from build123d import *

# Parameters (mm, degrees)
SKETCH_2_W           = 57
SKETCH_2_H           = 47.14
EXTRUDE_1_DEPTH      = 100
SKETCH_3_R           = 17.5
EXTRUDE_2_DEPTH      = 2
SKETCH_4_R           = 5
EXTRUDE_3_DEPTH      = 22
SKETCH_5_W           = 15.396782634
SKETCH_5_H           = 5.477116352
CUT_EXTRUDE_1_DEPTH  = 20
SKETCH_7_R           = 10
CUT_EXTRUDE_2_DEPTH  = 95
SKETCH_8_R           = 2.5
CUT_EXTRUDE_3_DEPTH  = 90
SKETCH_9_OUTSIDE_W   = 87.878
SKETCH_9_OUTSIDE_H   = 78.018
SKETCH_9_OUTSIDE_W_2 = 55
SKETCH_9_OUTSIDE_H_2 = 47.14
CUT_EXTRUDE_4_DEPTH  = 80
CUT_EXTRUDE_5_DEPTH  = 40
CUT_EXTRUDE_6_DEPTH  = 20
SKETCH_12_R          = 2
CUT_EXTRUDE_7_DEPTH  = 4


with BuildPart() as part:
    # 草图2 → 凸台-拉伸1 (new body)
    with BuildSketch(Plane.XY):
        Rectangle(SKETCH_2_W, SKETCH_2_H)
    extrude(amount=EXTRUDE_1_DEPTH)

    # 草图3 → 凸台-拉伸2 (add)
    with BuildSketch(Plane.XY.offset(100)):
        Circle(SKETCH_3_R)
    extrude(amount=EXTRUDE_2_DEPTH)

    # 草图4 → 凸台-拉伸3 (add)
    with BuildSketch(Plane.XY.offset(102)):
        Circle(SKETCH_4_R)
    extrude(amount=EXTRUDE_3_DEPTH)

    # 草图5 → 切除-拉伸1 (cut)
    with BuildSketch(Plane.XY.offset(124)):
        with Locations((0.517283211, -5.738558176)):
            Rectangle(SKETCH_5_W, SKETCH_5_H)
    extrude(amount=-CUT_EXTRUDE_1_DEPTH, mode=Mode.SUBTRACT)

    # 草图7 → 切除-拉伸2 (cut)
    with BuildSketch(Plane(origin=(0, 0, 0), x_dir=(-1, 0, 0), z_dir=(0, 0, -1))):
        with Locations((28.5, 23.57)):
            Circle(SKETCH_7_R)
        with Locations((28.5, -23.57)):
            Circle(SKETCH_7_R)
        with Locations((-28.5, -23.57)):
            Circle(SKETCH_7_R)
        with Locations((-28.5, 23.57)):
            Circle(SKETCH_7_R)
    extrude(amount=-CUT_EXTRUDE_2_DEPTH, mode=Mode.SUBTRACT)

    # 草图8 → 切除-拉伸3 (cut)
    with BuildSketch(Plane.XY.offset(100)):
        with Locations((-24.5, 19.57)):
            Circle(SKETCH_8_R)
        with Locations((24.5, 19.57)):
            Circle(SKETCH_8_R)
        with Locations((24.5, -19.57)):
            Circle(SKETCH_8_R)
        with Locations((-24.5, -19.57)):
            Circle(SKETCH_8_R)
    extrude(amount=-CUT_EXTRUDE_3_DEPTH, mode=Mode.SUBTRACT)

    # 草图9 outside → 切除-拉伸4 (cut)
    with BuildSketch(Plane(origin=(0, 0, 0), x_dir=(-1, 0, 0), z_dir=(0, 0, -1))):
        Rectangle(SKETCH_9_OUTSIDE_W, SKETCH_9_OUTSIDE_H)
        Rectangle(SKETCH_9_OUTSIDE_W_2, SKETCH_9_OUTSIDE_H_2, mode=Mode.SUBTRACT)
    extrude(amount=-CUT_EXTRUDE_4_DEPTH, mode=Mode.SUBTRACT)

    # 草图10 → 切除-拉伸5 (cut)
    with BuildSketch(Plane(origin=(0, 0, 0), x_dir=(-1, 0, 0), z_dir=(0, 0, -1))):
        with BuildLine():
            Line((-27.5, 13.620125629), (-27.5, -13.620125629))
            ThreePointArc((-27.5, -13.620125629), (-21.083801513, -16.861796068), (-18.5, -23.57))
            Line((-18.5, -23.57), (18.5, -23.57))
            ThreePointArc((18.5, -23.57), (21.083801513, -16.861796068), (27.5, -13.620125629))
            Line((27.5, -13.620125629), (27.5, 13.620125629))
            ThreePointArc((27.5, 13.620125629), (21.083801513, 16.861796068), (18.5, 23.57))
            Line((18.5, 23.57), (-18.5, 23.57))
            ThreePointArc((-18.5, 23.57), (-21.083801513, 16.861796068), (-27.5, 13.620125629))
        make_face()
        with BuildLine():
            Line((-27, 13.177695155), (-27, -13.177695155))
            ThreePointArc((-27, -13.177695155), (-20.728707305, -16.509050358), (-18.011911518, -23.07))
            Line((-18.011911518, -23.07), (18.011911518, -23.07))
            ThreePointArc((18.011911518, -23.07), (20.728707305, -16.509050358), (27, -13.177695155))
            Line((27, -13.177695155), (27, 13.177695155))
            ThreePointArc((27, 13.177695155), (20.728707305, 16.509050358), (18.011911518, 23.07))
            Line((18.011911518, 23.07), (-18.011911518, 23.07))
            ThreePointArc((-18.011911518, 23.07), (-20.728707305, 16.509050358), (-27, 13.177695155))
        make_face(mode=Mode.SUBTRACT)
    extrude(amount=-CUT_EXTRUDE_5_DEPTH, mode=Mode.SUBTRACT)

    # 草图11 → 切除-拉伸6 (cut)
    with BuildSketch(Plane(origin=(0, 0, 0), x_dir=(-1, 0, 0), z_dir=(0, 0, -1))):
        with BuildLine():
            Line((-27, 13.177695155), (-27, -13.177695155))
            ThreePointArc((-27, -13.177695155), (-20.728707305, -16.509050358), (-18.011911518, -23.07))
            Line((-18.011911518, -23.07), (18.011911518, -23.07))
            ThreePointArc((18.011911518, -23.07), (20.728707305, -16.509050358), (27, -13.177695155))
            Line((27, -13.177695155), (27, 13.177695155))
            ThreePointArc((27, 13.177695155), (20.728707305, 16.509050358), (18.011911518, 23.07))
            Line((18.011911518, 23.07), (-18.011911518, 23.07))
            ThreePointArc((-18.011911518, 23.07), (-20.728707305, 16.509050358), (-27, 13.177695155))
        make_face()
        with BuildLine():
            Line((17.54554885, 22.57), (-17.54554885, 22.57))
            ThreePointArc((-17.54554885, 22.57), (-20.373123341, 16.156911861), (-26.5, 12.753346174))
            Line((-26.5, 12.753346174), (-26.5, -12.753346174))
            ThreePointArc((-26.5, -12.753346174), (-20.373123341, -16.156911861), (-17.54554885, -22.57))
            Line((-17.54554885, -22.57), (17.54554885, -22.57))
            ThreePointArc((17.54554885, -22.57), (20.373123341, -16.156911861), (26.5, -12.753346174))
            Line((26.5, -12.753346174), (26.5, 12.753346174))
            ThreePointArc((26.5, 12.753346174), (20.373123341, 16.156911861), (17.54554885, 22.57))
        make_face(mode=Mode.SUBTRACT)
    extrude(amount=-CUT_EXTRUDE_6_DEPTH, mode=Mode.SUBTRACT)

    # 草图12 → 切除-拉伸7 (cut)
    with BuildSketch(Plane.XY.offset(100)):
        with Locations((-24.5, 13.5)):
            Circle(SKETCH_12_R)
        with Locations((-24.5, -13.5)):
            Circle(SKETCH_12_R)
        with Locations((24.5, -13.5)):
            Circle(SKETCH_12_R)
        with Locations((24.5, 13.5)):
            Circle(SKETCH_12_R)
    extrude(amount=-CUT_EXTRUDE_7_DEPTH, mode=Mode.SUBTRACT)


solid = part.part
Read the model definition and answer for the solid it produces. Units are mm, in the model's axes. A direction names the side the tool comes from. Give positions to 0.01 mm unless a question says otherwise; leave off trailing zeros. Write each loop counter-clockwise with the first axis right and the second up, starting at its lowest first coordinate (ties: lowest second). Pieces come first, ordered by that corner, then holes. Notation, with made-up numbers: (85, -3) - (114, -3) arc R23 ccw to (114, 31) - close; hole circle Ø4 at (-24.75, -38.5). An arc over 180 degrees is marked (long way). Return JSON: item names as keys, results as strings.
Q1. A cutting plane is placed at D-D, the plane z = 75. Determine the outline of the cut face in (x, y).
Reply:
{"outline": "(-27.5, -13.62) arc R10 cw to (-18.5, -23.57) - (18.5, -23.57) arc R10 cw to (27.5, -13.62) - (27.5, 13.62) arc R10 cw to (18.5, 23.57) - (-18.5, 23.57) arc R10 cw to (-27.5, 13.62) - close"}
Q2. A cutting plane is placed at C-C, the plane x = 0. Determine the outline of the cut face in (y, z).
Reply:
{"outline": "(-23.57, 40) - (-23.07, 40) - (-23.07, 20) - (-22.57, 20) - (-22.57, 0) - (22.57, 0) - (22.57, 20) - (23.07, 20) - (23.07, 40) - (23.57, 40) - (23.57, 100) - (17.5, 100) - (17.5, 102) - (5, 102) - (5, 124) - (-3, 124) - (-3, 104) - (-5, 104) - (-5, 102) - (-17.5, 102) - (-17.5, 100) - (-23.57, 100) - close"}
Q3. Given P1, Ø3, axis at x = -24.5, y = -16, coming from the -Z side; P2, Ø4, axis at y = 0.5, z = 48.5, coming from the +X side; P3, Ø5, axis at x = -24.5, y = -13.5, coming from the +Z side; P4, Ø3, axis at x = 24.5, y = -19.57, coming from the +Z side, each flat-ended and moving along its own axis, determine where each tip first touches the part or whether it passes through.
Reply:
{"P1": "z = 40", "P2": "x = 27.5", "P3": "z = 100", "P4": "through"}
Q4. A cutting plane is placed at A-A, the plane x = -25. Count the separate pieces of the cut face and the enclosed holes in it, and give its area (3 significant figures).
Reply:
{"separate pieces": "3", "enclosed holes": "0", "area": "2,790 mm²"}
Q5. Consider line 1 along Y through (x, z) = (-24.5, 96.8); line 2 along X through (y, z) = (-19, 98); line 3 along X through (y, z) = (13, 98). Determine where each line is inside the solid, lowest interval first. Write a range as [from, to].
Reply:
{"line 1": "[-23.57, -22.07], [-17.07, -15.5], [-11.5, 11.5], [15.5, 17.07], [22.07, 23.57]", "line 2": "[-28.5, -26.93], [-22.07, 22.07], [26.93, 28.5]", "line 3": "[-28.5, -26.44], [-22.56, 22.56], [26.44, 28.5]"}
Q6. For a pull along X with two mould halves and no side action, classify faces 1 (the face through (24.17, 22.05, 97.54)), 2 (the face through (22, 18, 95)), 3 (the face through (-20.661, -16.584, 29.86)) as released by +X, released by -X, zero draft, split by the parting line, or undercut.
Reply:
{"face 1": "undercut", "face 2": "zero draft", "face 3": "released by -X"}
Q7. A cutting plane is placed at B-B, the plane y = 19.57. Determine the outline of the cut face in (x, z).
Reply:
{"outline": "(-28.5, 95) - (-27, 95) - (-27, 100) - (-28.5, 100) - close; (-22, 95) - (-19.33, 95) - (-19.33, 40) - (-18.79, 40) - (-18.79, 20) - (-18.25, 20) - (-18.25, 0) - (18.25, 0) - (18.25, 20) - (18.79, 20) - (18.79, 40) - (19.33, 40) - (19.33, 95) - (22, 95) - (22, 100) - (-22, 100) - close; (27, 95) - (28.5, 95) - (28.5, 100) - (27, 100) - close"}
Q8. For faces 4 (the face through (20.661, 16.584, 29.86)), 5 (the face through (-25.974, -12.148, 98.028)), 6 (the face through (-21.51, -16.42, 67.11)), 7 (the face through (26.5, 0, 10)), 8 (the face through (-27, 0, 30)), determine the directions among +Z, -Z, +X, -X, +Y, -Y from which every point of the face is accessible in a straight line to the end or side of a thin tool.
Reply:
{"face 4": "-Z, +X, +Y", "face 5": "+Z", "face 6": "-Z, -X, -Y", "face 7": "-Z, +X, +Y, -Y", "face 8": "-Z, -X, +Y, -Y"}
